Source: CAD feature listing. Evaluate the final solid. Frame: model axes, mm. Face numbers are marked on the shaded views. A direction names the side the tool comes from. Give positions to 0.01 mm unless a question says otherwise; leave off trailing zeros. Order: outer loops, then holes, each group sorted by start corner. A loop starts at its lowest first (then second) coordinate and runs counter-clockwise, first axis right, second up. Notation, with made-up numbers: (-4, 59.25) - (47, 59.25) arc R25 cw to (47, 79.25) - close; hole circle Ø6 at (-21, 2.25). An arc over 180 degrees is marked (long way). Answer as CSV lines item,"result".
```python
from build123d import *

# Parameters (mm, degrees)
SKETCH_1_R          = 1.025
SKETCH_1_R_2        = 10.25
EXTRUDE_2_DEPTH     = 5
SKETCH_2_W          = 40
SKETCH_2_H          = 5
EXTRUDE_3_DEPTH     = 50
CUT_EXTRUDE_1_REACH = 77.166
SKETCH_3_R          = 1.525
EXTRUDE_4_DEPTH     = 3
EXTRUDE_5_DEPTH     = 3


with BuildPart() as part:
    # 草图1 → 凸台-拉伸2 (new body)
    with BuildSketch(Plane(origin=(0, 0, 0), x_dir=(1, 0, 0), z_dir=(0, 1, 0))):
        with BuildLine():
            ThreePointArc((0, 20), (5.857864376, 5.857864376), (20, 0))
            ThreePointArc((20, 0), (34.142135624, 5.857864376), (40, 20))
            Line((40, 20), (40, 40))
            Line((40, 40), (0, 40))
            Line((0, 40), (0, 20))
        make_face()
        with Locations(Location((7.009618943, 12.5, 0), (0, 0, 270))):
            Circle(SKETCH_1_R, mode=Mode.SUBTRACT)
        with Locations(Location((20, 5, 0), (0, 0, 270))):
            Circle(SKETCH_1_R, mode=Mode.SUBTRACT)
        with Locations(Location((32.990381057, 12.5, 0), (0, 0, 270))):
            Circle(SKETCH_1_R, mode=Mode.SUBTRACT)
        with Locations(Location((7.009618943, 27.5, 0), (0, 0, 270))):
            Circle(SKETCH_1_R, mode=Mode.SUBTRACT)
        with Locations(Location((20, 20, 0), (0, 0, 270))):
            Circle(SKETCH_1_R_2, mode=Mode.SUBTRACT)
        with Locations(Location((32.990381057, 27.5, 0), (0, 0, 270))):
            Circle(SKETCH_1_R, mode=Mode.SUBTRACT)
        with Locations(Location((20, 35, 0), (0, 0, 270))):
            Circle(SKETCH_1_R, mode=Mode.SUBTRACT)
    extrude(amount=EXTRUDE_2_DEPTH)

    # 草图2 → 凸台-拉伸3 (add)
    with BuildSketch(Plane(origin=(0, 5, 0), x_dir=(1, 0, 0), z_dir=(0, 1, 0))):
        with Locations((20, 42.5)):
            Rectangle(SKETCH_2_W, SKETCH_2_H)
    extrude(amount=-EXTRUDE_3_DEPTH)

    # 草图3 → 切除-拉伸1 (cut, up to next)
    with BuildSketch(Plane(origin=(0, 0, -45), x_dir=(-1, 0, 0), z_dir=(0, 0, -1)), mode=Mode.PRIVATE) as cut_extrude_1_sk1:
        with Locations((-7, -12)):
            Circle(SKETCH_3_R)
    cut_extrude_1_tool1 = extrude(cut_extrude_1_sk1.sketch, amount=-CUT_EXTRUDE_1_REACH, mode=Mode.PRIVATE) & part.part
    # 草图3 → 切除-拉伸1 (cut, up to next)
    with BuildSketch(Plane(origin=(0, 0, -45), x_dir=(-1, 0, 0), z_dir=(0, 0, -1)), mode=Mode.PRIVATE) as cut_extrude_1_sk2:
        with Locations((-7, -38)):
            Circle(SKETCH_3_R)
    cut_extrude_1_tool2 = extrude(cut_extrude_1_sk2.sketch, amount=-CUT_EXTRUDE_1_REACH, mode=Mode.PRIVATE) & part.part
    # 草图3 → 切除-拉伸1 (cut, up to next)
    with BuildSketch(Plane(origin=(0, 0, -45), x_dir=(-1, 0, 0), z_dir=(0, 0, -1)), mode=Mode.PRIVATE) as cut_extrude_1_sk3:
        with Locations((-33, -38)):
            Circle(SKETCH_3_R)
    cut_extrude_1_tool3 = extrude(cut_extrude_1_sk3.sketch, amount=-CUT_EXTRUDE_1_REACH, mode=Mode.PRIVATE) & part.part
    # 草图3 → 切除-拉伸1 (cut, up to next)
    with BuildSketch(Plane(origin=(0, 0, -45), x_dir=(-1, 0, 0), z_dir=(0, 0, -1)), mode=Mode.PRIVATE) as cut_extrude_1_sk4:
        with Locations((-33, -12)):
            Circle(SKETCH_3_R)
    cut_extrude_1_tool4 = extrude(cut_extrude_1_sk4.sketch, amount=-CUT_EXTRUDE_1_REACH, mode=Mode.PRIVATE) & part.part
    add(cut_extrude_1_tool1.solids().sort_by_distance((7, -12, -45))[0], mode=Mode.SUBTRACT)
    add(cut_extrude_1_tool2.solids().sort_by_distance((7, -38, -45))[0], mode=Mode.SUBTRACT)
    add(cut_extrude_1_tool3.solids().sort_by_distance((33, -38, -45))[0], mode=Mode.SUBTRACT)
    add(cut_extrude_1_tool4.solids().sort_by_distance((33, -12, -45))[0], mode=Mode.SUBTRACT)

    # 草图4 → 凸台-拉伸4 (add)
    with BuildSketch(Plane.ZY):
        Polygon((-30, 0), (-40, 0), (-40, -10), align=None)
    extrude(amount=-EXTRUDE_4_DEPTH)

    # 草图5 → 凸台-拉伸5 (add)
    with BuildSketch(Plane(origin=(40, 0, 0), x_dir=(0, 0, -1), z_dir=(1, 0, 0))):
        Polygon((40, -10), (40, 0), (30, 0), align=None)
    extrude(amount=-EXTRUDE_5_DEPTH)


solid = part.part
```
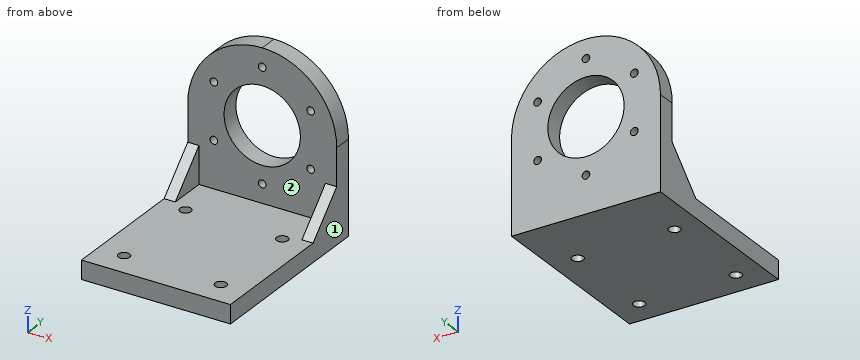
(1) Cut plane C-C (x = 17). Return loops of the section in (y, z).
Completed:
outline,"(-45, -45) - (5, -45) - (5, -29.8) - (0, -29.8) - (0, -40) - (-45, -40) - close; (0, -10.2) - (5, -10.2) - (5, -0.23) - (0, -0.23) - close"
(2) Cut plane D-D (z = -12.5). Return loops of the section in (x, y).
Completed:
outline,"(1.46, 0) - (5.98, 0) - (5.98, 5) - (1.46, 5) - close; (8.03, 0) - (13.01, 0) - (13.01, 5) - (8.03, 5) - close; (26.99, 0) - (31.97, 0) - (31.97, 5) - (26.99, 5) - close; (34.02, 0) - (38.54, 0) - (38.54, 5) - (34.02, 5) - close"
(3) Cut plane B-B (y = -12). Return loops of the section in (x, z) (3 decimals).
Completed:
outline,"(0, -45) - (5.475, -45) - (5.475, -40) - (0, -40) - close; (8.525, -45) - (31.475, -45) - (31.475, -40) - (8.525, -40) - close; (34.525, -45) - (40, -45) - (40, -40) - (34.525, -40) - close"
(4) Cut plane A-A (z = -35). Return loops of the section in (x, y) (3 decimals), then the cut area to 3 significant figures.
Completed:
outline,"(0, -5) - (3, -5) - (3, 0) - (18.975, 0) - (18.975, 5) - (0, 5) - close; (21.025, 0) - (37, 0) - (37, -5) - (40, -5) - (40, 5) - (21.025, 5) - close"
area,"220 mm²"
(5) Access query for the marked faces 1 and 2. Directions: +Z, -Z, +X, -X, +Y, -Y. A direction counts if a zero-diameter tool reaches every point of the face in a straight line with its end or side. Return the directions, or none.
Completed:
face 1,"+Z, -Z, +X, +Y, -Y"
face 2,"+Z, -Y"
(6) Ray query, line 1 (X direction, y = 1.7, z = -27.5); line 2 (Z direction, x = 15, y = -21.5); line 3 (Y direction, x = 26, z = -28.5). Return the intervals inside material, ascending. Write a range as from..to.
Completed:
line 1,"0..5.98, 8.03..13.01, 26.99..31.97, 34.02..40"
line 2,"-45..-40"
line 3,"0..5"
(7) Contact query for flat-ended pins moving along their axis: pin 1 (6 mm diameter, centred on x = 8, y = -17.5, fed in from +Z); pin 2 (2.5 mm diameter, centred on x = 7.01, z = -27.5, fed in from -Y). Output: stop coordinate, or through.
Completed:
pin 1,"z = -40"
pin 2,"y = 0"
